Geometry check sheet. Reference: the model listing, model coordinates, mm. Face numbers are marked on the shaded views. A direction names the side the tool comes from. Round coordinates to 2 decimals unless told otherwise and drop trailing zeros. Order: outer loops, then holes, each group sorted by start corner. A loop starts at its lowest first (then second) coordinate and runs counter-clockwise, first axis right, second up. Notation, with made-up numbers: M 56,-17.5 L 94,-17.5 A29 cw 94,13.5 Z; hole C 55,48 d1. An arc over 180 degrees is marked long. Answer as a JSON object with one key per item and string values. Group by question number.
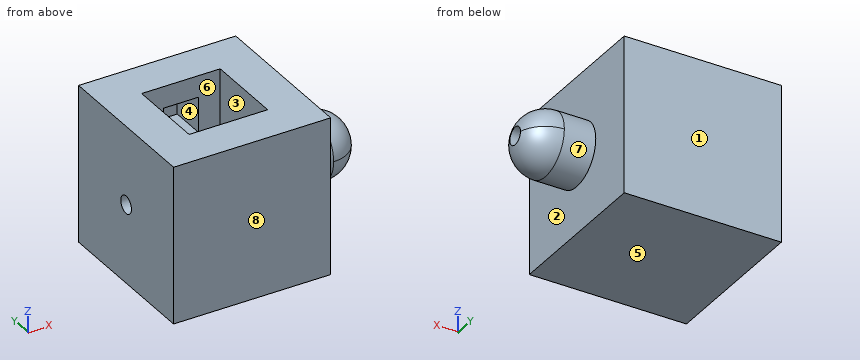
```python
from build123d import *

# Parameters (mm, degrees)
F0_W           = 5
F0_H           = 5
F2_DEPTH       = 5
F3_W           = 2.5
F3_H           = 2.5
F4_DEPTH       = 2.5
F5_W           = 1.125
F5_H           = 1.125
F6_DEPTH       = 1.125
F7_R           = 1
F8_DEPTH       = 1
F10_ANGLE      = 180
F11_R          = 0.2796205341
F12_DEPTH      = 25.4
F13_DEPTH      = 2
F13_DEPTH_BACK = 5


# Not quite as in the source:
# - the program builds the solid bodies; features that only make, move or delete a surface that nothing else refers to are left out


with BuildPart() as f2:
    # F0 (on Top) → F2 (new body)
    with BuildSketch(Plane.XY):
        with Locations((2.5, -2.5)):
            Rectangle(F0_W, F0_H)
    extrude(amount=F2_DEPTH)

    # F3 (on face) → F4 (cut)
    with BuildSketch(Plane.XY.offset(5)):
        with Locations((2.5, -2.5)):
            Rectangle(F3_W, F3_H)
    extrude(amount=-F4_DEPTH, mode=Mode.SUBTRACT)

    # F5 (on face) → F6 (cut)
    with BuildSketch(Plane.XZ.offset(1.25)):
        with Locations((2.5, 3.75)):
            Rectangle(F5_W, F5_H)
    extrude(amount=-F6_DEPTH, mode=Mode.SUBTRACT)

    # F7 (on face) → F8 (join)
    with BuildSketch(Plane.YZ.offset(5)):
        with Locations((-2.5, 2.5)):
            Circle(F7_R)
    extrude(amount=F8_DEPTH)

    # F9 (on face) → F10 (revolve)
    with BuildSketch(Plane.YZ.offset(6)):
        with BuildLine():
            ThreePointArc((-1.5, 2.5), (-1.7928932188, 3.2071067812), (-2.5, 3.5))
            Line((-2.5, 3.5), (-2.5, 1.5))
            ThreePointArc((-2.5, 1.5), (-1.7928932188, 1.7928932188), (-1.5, 2.5))
        make_face()
    revolve(axis=Axis((6, -2.5, 2.5), (0, 0, -1)), revolution_arc=F10_ANGLE)

    # F11 (on face) → F12 (cut)
    with BuildSketch(Plane.YZ.offset(5)):
        with Locations((-2.5, 2.5)):
            Circle(F11_R)
    extrude(amount=F12_DEPTH, mode=Mode.SUBTRACT)

    # F11 (on face) → F13 (cut, two sides)
    with BuildSketch(Plane.YZ.offset(5)) as f13_sk:
        with Locations((-2.5, 2.5)):
            Circle(F11_R)
    extrude(amount=F13_DEPTH, mode=Mode.SUBTRACT)
    extrude(f13_sk.sketch, amount=-F13_DEPTH_BACK, mode=Mode.SUBTRACT)


solid = f2.part
```
1) Go/stop test with a flat-tipped pin: P1, Ø0.8, axis at y = -2.5, z = 3.5, coming from the +X side. Record where the tip stops, or that it passes through.
2) Sectioned sample at C-C (x = 6.75). Record the boundary of the cut face in (y, z).
3) Thickness scan on line 1 along Y through (x, z) = (1.5, 3.4); line 2 along Z through (x, y) = (5.65, -2.5); line 3 along Y through (x, z) = (5.65, 2.5). Record the ranges inside material, lowest first. Write a range as [from, to].
4) Sectioned sample at A-A (y = -2.5). Record the boundary of the cut face in (x, z), then the cut area to 3 significant figures.
5) Sectioned sample at D-D (z = 0.65). Record the boundary of the cut face in (x, y), then the cut area to 3 significant figures.
6) Sectioned sample at B-B (z = 4.4). Record the boundary of the cut face in (x, y).
7) Set-up check for the marked faces 4, 5, 6, 7 and 8: record each of +Z, -Z, +X, -X, +Y, -Y from which the full face is reachable in a straight line by a thin tool's end or side.
8) Release check for a two-part mould opening along X. For the marked faces 1, 2 and 3 record: +X half, -X half, draft (parallel to the pull), parting line (faces both ways), or undercut.
Final values:
{
 "1": {"P1": "stops at x = 6.8"},
 "2": {"outline": "C -2.5,2.5 d1.32; hole C -2.5,2.5 d0.56"},
 "3": {"line 1": "y = [-5, -3.75], [-1.25, 0]", "line 2": "z = [1.5, 2.22], [2.78, 3.5]", "line 3": "y = [-3.5, -2.78], [-2.22, -1.5]"},
 "4": {"outline": "M 0,0 L 5,0 L 5,1.5 L 6,1.5 A1 ccw 6.96,2.22 L 0,2.22 Z; M 0,2.78 L 1.25,2.78 L 1.25,5 L 0,5 Z; M 3.75,2.78 L 6.96,2.78 A1 ccw 6,3.5 L 5,3.5 L 5,5 L 3.75,5 Z", "area": "19.1 mm^2"},
 "5": {"outline": "M 0,-5 L 5,-5 L 5,0 L 0,0 Z", "area": "25.0 mm^2"},
 "6": {"outline": "M 0,-5 L 5,-5 L 5,0 L 0,0 Z; hole M 1.25,-3.75 L 3.75,-3.75 L 3.75,-1.25 L 1.25,-1.25 Z"},
 "7": {"face 4": "none", "face 5": "-Z, +X, -X, +Y, -Y", "face 6": "+Z", "face 7": "+X", "face 8": "+Z, -Z, +X, -X, -Y"},
 "8": {"face 1": "draft", "face 2": "+X half", "face 3": "undercut"}
}
